Verification items for the finished model (mm, model axes). A direction names the side the tool comes from. Coordinates: 2 decimals unless noted, no trailing zeros. Order: outer loops, then holes, each group sorted by start corner. A loop starts at its lowest first (then second) coordinate and runs counter-clockwise, first axis right, second up. Notation, with made-up numbers: M -37,41.5 L -15,41.5 A16 ccw -15,50.5 Z; hole C 72.5,17.25 d3. An arc over 180 degrees is marked long. Write item = value, one per line.
```python
from build123d import *

# Parameters (mm, degrees)
SKETCH1_R           = 3
SKETCH1_R_2         = 2
BOSS_EXTRUDE1_DEPTH = 2.05
CIRPATTERN7_COUNT   = 6
BOSS_EXTRUDE4_DEPTH = 4.1
CIRPATTERN8_COUNT   = 6
FILLET3_R           = 0.5


with BuildPart() as part:
    # Sketch1 → Boss-Extrude1 (new, symmetric)
    with BuildSketch(Plane(origin=(0, 0, 0), x_dir=(1, 0, 0), z_dir=(0, 1, 0))):
        with Locations(Location((0, 8.4, 0), (0, 0, 270))):
            Circle(SKETCH1_R)
        with Locations(Location((0, 8.4, 0), (0, 0, 270))):
            Circle(SKETCH1_R_2, mode=Mode.SUBTRACT)
    extrude(amount=BOSS_EXTRUDE1_DEPTH, both=True)


with BuildPart() as cirpattern7_1:
    # CirPattern7: pattern copy
    add(part.part.rotate(Axis((0, 0, 0), (0, 1, 0)), 1 * 360 / CIRPATTERN7_COUNT))


with BuildPart() as cirpattern7_2:
    # CirPattern7: pattern copy
    add(part.part.rotate(Axis((0, 0, 0), (0, 1, 0)), 2 * 360 / CIRPATTERN7_COUNT))


with BuildPart() as cirpattern7_3:
    # CirPattern7: pattern copy
    add(part.part.rotate(Axis((0, 0, 0), (0, 1, 0)), 3 * 360 / CIRPATTERN7_COUNT))


with BuildPart() as cirpattern7_4:
    # CirPattern7: pattern copy
    add(part.part.rotate(Axis((0, 0, 0), (0, 1, 0)), 4 * 360 / CIRPATTERN7_COUNT))


with BuildPart() as cirpattern7_5:
    # CirPattern7: pattern copy
    add(part.part.rotate(Axis((0, 0, 0), (0, 1, 0)), 5 * 360 / CIRPATTERN7_COUNT))


with BuildPart() as part_1:
    add(part.part)

    # Sketch5 → Boss-Extrude4 (add)
    with BuildSketch(Plane(origin=(0, 2.05, 0), x_dir=(1, 0, 0), z_dir=(0, 1, 0))):
        with BuildLine():
            Line((-4.384036917, 5.002849702), (-2.140576475, 6.298112192))
            ThreePointArc((-2.140576475, 6.298112192), (-2.598076211, 6.9), (-2.890576475, 7.597150298))
            Line((-2.890576475, 7.597150298), (-5.134036917, 6.301887808))
            ThreePointArc((-5.134036917, 6.301887808), (-4.67653718, 5.7), (-4.384036917, 5.002849702))
        make_face()
    extrude(amount=-BOSS_EXTRUDE4_DEPTH)


with BuildPart() as cirpattern8_1:
    # CirPattern8: pattern copy
    add(part_1.part.rotate(Axis((0, 0, 0), (0, 1, 0)), 1 * 360 / CIRPATTERN8_COUNT))


with BuildPart() as cirpattern8_2:
    # CirPattern8: pattern copy
    add(part_1.part.rotate(Axis((0, 0, 0), (0, 1, 0)), 2 * 360 / CIRPATTERN8_COUNT))


with BuildPart() as cirpattern8_3:
    # CirPattern8: pattern copy
    add(part_1.part.rotate(Axis((0, 0, 0), (0, 1, 0)), 3 * 360 / CIRPATTERN8_COUNT))


with BuildPart() as cirpattern8_4:
    # CirPattern8: pattern copy
    add(part_1.part.rotate(Axis((0, 0, 0), (0, 1, 0)), 4 * 360 / CIRPATTERN8_COUNT))


with BuildPart() as cirpattern8_5:
    # CirPattern8: pattern copy
    add(part_1.part.rotate(Axis((0, 0, 0), (0, 1, 0)), 5 * 360 / CIRPATTERN8_COUNT))


with BuildPart() as cirpattern8_4_1:
    add(cirpattern8_4.part)

    # Combine1: read off the stored shape, not the designer's step
    # Combine1: union CirPattern7_5, CirPattern7_3, CirPattern7_2, CirPattern7_1, part, CirPattern8_5, CirPattern8_3, CirPattern8_2, CirPattern8_1, CirPattern7_4
    add(cirpattern7_5.part)
    add(cirpattern7_3.part)
    add(cirpattern7_2.part)
    add(cirpattern7_1.part)
    add(part_1.part)
    add(cirpattern8_5.part)
    add(cirpattern8_3.part)
    add(cirpattern8_2.part)
    add(cirpattern8_1.part)
    add(cirpattern7_4.part)

    # Fillet3
    fillet3_edges = [cirpattern8_4_1.edges().sort_by_distance(p)[0] for p in [
        (-8.024613392, 0, -1.29526249),
        (-4.384036917, 0, -5.002849702),
        (-8.024613392, 0, 1.29526249),
        (-6.524613392, 0, -1.29526249),
        (-6.524613392, 0, 1.29526249),
        (-5.134036917, 0, 6.301887808),
        (-2.890576475, 0, 7.597150298),
        (-4.384036917, 0, 5.002849702),
        (-2.140576475, 0, 6.298112192),
        (2.890576475, 0, 7.597150298),
        (5.134036917, 0, 6.301887808),
        (2.140576475, 0, 6.298112192),
        (4.384036917, 0, 5.002849702),
        (8.024613392, 0, 1.29526249),
        (8.024613392, 0, -1.29526249),
        (6.524613392, 0, 1.29526249),
        (6.524613392, 0, -1.29526249),
        (5.134036917, 0, -6.301887808),
        (2.890576475, 0, -7.597150298),
        (4.384036917, 0, -5.002849702),
        (2.140576475, 0, -6.298112192),
        (-2.890576475, 0, -7.597150298),
        (-5.134036917, 0, -6.301887808),
        (-2.140576475, 0, -6.298112192),
    ]]
    fillet(fillet3_edges, radius=FILLET3_R)


solid = cirpattern8_4_1.part
```
Item 1: Sectioned sample at D-D, the plane y = -1.8. Give the number of separate pieces and of enclosed holes in the cut face, then the cut area to 3 significant figures.
Report:
separate_pieces = 1
enclosed_holes = 7
area = 117 mm^2
Item 2: Tool access check on faces 1 (the flat face through (-8.025, 0, 0)), 2 (the cylindrical face through (0, 0, 5.4)). Record the directions out of +Z, -Z, +X, -X, +Y, -Y that give a thin tool (end or side, any length) a straight path to the whole face; none if there is none.
Report:
face_1 = -X, +Y, -Y
face_2 = +Y, -Y
Item 3: Scan lines: L1, parallel to X at y = 0.15, z = -4.2; L2, parallel to Z at x = 0.75, y = 1.7; L3, parallel to Z at x = -8.75, y = 0.7. Record each from-to range of solid material in increasing order. Write a range as from..to.
Report:
L1 = -10.27..-9.27, -5.27..-4.27, 4.27..5.27, 9.27..10.27
L2 = -11.3..-10.25, -6.55..-5.5, 5.5..6.55, 10.25..11.3
L3 = -6.81..-5.55, -2.85..-1.59, 1.59..2.85, 5.55..6.81
Item 4: Sectioned sample at B-B, the plane x = 0. Enter the section's corners in (y, z).
Report:
outline = M -2.05,-11.4 L 2.05,-11.4 L 2.05,-10.4 L -2.05,-10.4 Z; M -2.05,-6.4 L 2.05,-6.4 L 2.05,-5.4 L -2.05,-5.4 Z; M -2.05,5.4 L 2.05,5.4 L 2.05,6.4 L -2.05,6.4 Z; M -2.05,10.4 L 2.05,10.4 L 2.05,11.4 L -2.05,11.4 Z
Item 5: Sectioned sample at A-A, the plane z = -8.4. Enter the section's corners in (x, y), then the cut area to 3 significant figures.
Report:
outline = M -3,-2.05 L -2,-2.05 L -2,2.05 L -3,2.05 Z; M 2,-2.05 L 3,-2.05 L 3,2.05 L 2,2.05 Z
area = 8.20 mm^2
Item 6: Sectioned sample at C-C, the plane z = 4.2. Enter the section's corners in (x, y), then the cut area to 3 significant figures.
Report:
outline = M -10.27,-2.05 L -9.27,-2.05 L -9.27,2.05 L -10.27,2.05 Z; M -5.27,-2.05 L -4.27,-2.05 L -4.27,2.05 L -5.27,2.05 Z; M 4.27,-2.05 L 5.27,-2.05 L 5.27,2.05 L 4.27,2.05 Z; M 9.27,-2.05 L 10.27,-2.05 L 10.27,2.05 L 9.27,2.05 Z
area = 16.4 mm^2
Item 7: Gauge pin test, flat ends, axial feed: pin 1 (0.6 mm diameter, centred on y = 0, z = 0.5, fed in from -X); pin 2 (0.9 mm diameter, centred on y = 0.5, z = -0.5, fed in from +X) (3 decimals); pin 3 (1 mm diameter, centred on y = 1, z = -1, fed in from +X). Record the tip position at first contact, or that the pin passes through.
Report:
pin_1 = -8.02
pin_2 = 8.025
pin_3 = 8.58
Item 8: Release check for a two-part mould opening along Z. For faces 3 (the flat face through (-4.001, 0.029, -6.956)), 4 (the cylindrical face through (4.69, 0.03, 2.68)), 5 (the flat face through (-4.024, 0.029, 6.943)) record: pulls with the +Z half, pulls with the -Z half, needs draft (parallel to the pull), parting line crosses it, or undercut.
Report:
face_3 = pulls with the -Z half
face_4 = undercut
face_5 = pulls with the +Z half
